from build123d import *

# Parameters (mm, degrees)
CUT_EXTRUDE1_DEPTH       = 22.365860619
CUT_EXTRUDE1_DEPTH_BACK  = 22.365860619
SKETCH2_R                = 1.5
SKETCH3_W                = 9.16515139
SKETCH3_H                = 1.7
CUT_EXTRUDE2_DEPTH       = 21.310096204
FILLET1_R                = 0.4
BOSS_EXTRUDE1_START      = 19.2405
SKETCH4_R                = 6.5
SKETCH4_R_2              = 3
BOSS_EXTRUDE1_DEPTH      = 19.2405
CHAMFER1_SIZE            = 1.5
CHAMFER2_SIZE            = 0.5
FILLET2_R                = 0.5
CUT_EXTRUDE3_START       = -19.2405
CUT_EXTRUDE3_OUTLINE_R   = 7.963373885
CUT_EXTRUDE3_OUTLINE_R_2 = 3
CUT_EXTRUDE3_DEPTH       = 19.2405
SKETCH6_R                = 3.5
CUT_EXTRUDE4_DEPTH       = 10
CHAMFER3_SIZE            = 0.5
SKETCH7_R                = 10.7
CUT_EXTRUDE5_DEPTH       = 10
CUT_EXTRUDE6_START       = 5.5
CUT_EXTRUDE6_DEPTH       = 1.7
CHAMFER5_SIZE            = 1


# Read off the part's stored shape, not the designer's step: Cut-Extrude3
with BuildPart() as part:
    # Sketch1 → Revolve1 (revolve)
    with BuildSketch(Plane.XY, mode=Mode.PRIVATE) as revolve1_sk:
        Polygon((-12, 12.5), (0, 12.5), (6, 12.5), (6, 10), (6, 3), (-2, 3), (-2, 10.2), (-12, 10.2), align=None)
    revolve(revolve1_sk.sketch.rotate(Axis((88.99, 0, 0), (-1, 0, 0)), 90), axis=Axis((88.99, 0, 0), (-1, 0, 0)))

    # Sketch2 → Cut-Extrude1 (cut, two sides: drawn at the far end of the back side and taken through both)
    with BuildSketch(Plane(origin=(0, 0, 0), x_dir=(1, 0, 0), z_dir=(0, 1, 0)).offset(-CUT_EXTRUDE1_DEPTH_BACK)):
        with Locations(Location((3, 0, 0), (0, 0, 90))):
            Circle(SKETCH2_R)
    extrude(amount=CUT_EXTRUDE1_DEPTH + CUT_EXTRUDE1_DEPTH_BACK, mode=Mode.SUBTRACT)

    # Sketch3 → Cut-Extrude2 (cut, through all)
    with BuildSketch(Plane.ZY.offset(2)):
        with Locations((-4.582575695, 9.35)):
            Rectangle(SKETCH3_W, SKETCH3_H)
    extrude(amount=CUT_EXTRUDE2_DEPTH, mode=Mode.SUBTRACT)

    # Fillet1
    fillet1_edges = [part.edges().sort_by_distance(p)[0] for p in [
        (-7, 8.5, -5.638262144),
        (-7, 10.2, -7.22564876),
        (-7, 8.5, -9.16515139),
    ]]
    fillet(fillet1_edges, radius=FILLET1_R)

    # Sketch4 → Boss-Extrude1 (add)
    with BuildSketch(Plane.ZY.offset(2).offset(BOSS_EXTRUDE1_START)):
        Circle(SKETCH4_R)
        with Locations(Location((0, 0, 0), (0, 0, 180))):
            Circle(SKETCH4_R_2, mode=Mode.SUBTRACT)
    extrude(amount=-BOSS_EXTRUDE1_DEPTH)

    # Chamfer1
    chamfer1_edges = [part.edges().sort_by_distance(p)[0] for p in [
        (-21.2405, 0, -6.5),
        (-21.2405, 0, 3),
    ]]
    chamfer(chamfer1_edges, length=CHAMFER1_SIZE)

    # Chamfer2
    chamfer2_edges = [part.edges().sort_by_distance(p)[0] for p in [
        (6, 0, 3),
    ]]
    chamfer(chamfer2_edges, length=CHAMFER2_SIZE)

    # Fillet2
    # the kernel refuses this fillet: 0.5 mm, written as the material it adds along each edge
    with BuildSketch(Plane(origin=(-2, 0, 0), x_dir=(0, 0.7641509433962261, -0.6450374684517619), z_dir=(0, 0.6450374684517619, 0.7641509433962261))) as fillet2_piece_1:
        with BuildLine():
            CenterArc((10.2 - FILLET2_R, FILLET2_R), FILLET2_R, 270, 90)
            Line((10.2, FILLET2_R), (10.2, 0))
            Line((10.2, 0), (10.2 - FILLET2_R, 0))
        make_face()
    revolve(axis=Axis((-2, 0, 0), (-1, 0, 0)), revolution_arc=319.831515217)
    with BuildSketch(Plane(origin=(-2, 10.2, 0), x_dir=(0, -1, 0), z_dir=(0, 0, -1))) as fillet2_piece_2:
        with BuildLine():
            CenterArc((FILLET2_R, FILLET2_R), FILLET2_R, 180, 90)
            Line((0, FILLET2_R), (0, 0))
            Line((0, 0), (FILLET2_R, 0))
        make_face()
    extrude(amount=5.835237784)
    with BuildSketch(Plane(origin=(-2, 8.5, -8.988882022), x_dir=(0, 1, 0), z_dir=(0, 0, 1))) as fillet2_piece_3_section:
        with BuildLine():
            CenterArc((FILLET2_R, FILLET2_R), FILLET2_R, 180, 90)
            Line((0, FILLET2_R), (0, 0))
            Line((0, 0), (FILLET2_R, 0))
        make_face()
    fillet2_piece_3 = extrude(amount=2.151484856, mode=Mode.PRIVATE)
    fillet2_piece_3 = fillet2_piece_3 & Plane(origin=(-2.112337318, 0, 0), x_dir=(0, 0, -1), z_dir=(1, 0, 0)) * Cylinder(12.5, 7, mode=Mode.PRIVATE)
    add(fillet2_piece_3)
    with BuildSketch(Plane(origin=(-2, 8.1, -6.837397166), x_dir=(0, -0.7641509433962268, 0.6450374684517612), z_dir=(0, -0.6450374684517612, -0.7641509433962268))) as fillet2_piece_4:
        with BuildLine():
            CenterArc((0.4 + FILLET2_R, FILLET2_R), FILLET2_R, 180, 90)
            Line((0.4, FILLET2_R), (0.4, 0))
            Line((0.4, 0), (0.4 + FILLET2_R, 0))
        make_face()
    revolve(axis=Axis((-2, 8.1, -6.837397166), (-1, 0, 0)), revolution_arc=139.831515217)
    with BuildSketch(Plane(origin=(-2, 8.1, -8.988882022), x_dir=(0, -0.6813941617388248, 0.7319166594280009), z_dir=(0, 0.7319166594280009, 0.6813941617388248))) as fillet2_piece_5_section:
        with BuildLine():
            CenterArc((0.4 + FILLET2_R, -FILLET2_R), FILLET2_R, 90, 90)
            Line((0.4, -FILLET2_R), (0.4, 0))
            Line((0.4, 0), (0.4 + FILLET2_R, 0))
        make_face()
    fillet2_piece_5 = revolve(axis=Axis((-2, 8.1, -8.988882022), (1, 0, 0)), revolution_arc=227.047315948, mode=Mode.PRIVATE)
    fillet2_piece_5 = fillet2_piece_5 & Plane(origin=(-2.20433756, 0, 0), x_dir=(0, 0, -1), z_dir=(1, 0, 0)) * Cylinder(12.5, 4, mode=Mode.PRIVATE)
    add(fillet2_piece_5)
    with BuildSketch(Plane(origin=(-2, 10.6, -5.835237784), x_dir=(0, -0.8696656127523182, 0.49364128878785535), z_dir=(0, -0.49364128878785535, -0.8696656127523182))) as fillet2_piece_6_section:
        with BuildLine():
            CenterArc((0.4 + FILLET2_R, FILLET2_R), FILLET2_R, 180, 90)
            Line((0.4 + FILLET2_R, 0), (0.4, 0))
            Line((0.4, 0), (0.4, FILLET2_R))
        make_face()
    fillet2_piece_6 = revolve(axis=Axis((-2, 10.6, -5.835237784), (-1, 0, 0)), revolution_arc=330.419804772, mode=Mode.PRIVATE)
    fillet2_piece_6 = fillet2_piece_6 & Plane(origin=(-2.048284791, 0, 0), x_dir=(0, 0, -1), z_dir=(1, 0, 0)) * Cylinder(12.5, 4, mode=Mode.PRIVATE)
    add(fillet2_piece_6)
    with BuildSketch(Plane(origin=(-2, 0, 0), x_dir=(0, 0, 1), z_dir=(0, -1, 0))) as fillet2_piece_7:
        with BuildLine():
            CenterArc((6.5 + FILLET2_R, FILLET2_R), FILLET2_R, 180, 90)
            Line((6.5, FILLET2_R), (6.5, 0))
            Line((6.5, 0), (6.5 + FILLET2_R, 0))
        make_face()
    revolve(axis=Axis((-2, 0, 0), (-1, 0, 0)))

    # Cut-Extrude3 outline → Cut-Extrude3 (cut)
    with BuildSketch(Plane.ZY.offset(21.2405).offset(CUT_EXTRUDE3_START)):
        Circle(CUT_EXTRUDE3_OUTLINE_R)
        Circle(CUT_EXTRUDE3_OUTLINE_R_2, mode=Mode.SUBTRACT)
    extrude(amount=CUT_EXTRUDE3_DEPTH, mode=Mode.SUBTRACT)

    # Sketch6 → Cut-Extrude4 (cut)
    with BuildSketch(Plane(origin=(6, 0, 0), x_dir=(0, 0, -1), z_dir=(1, 0, 0))):
        Circle(SKETCH6_R)
    extrude(amount=-CUT_EXTRUDE4_DEPTH, mode=Mode.SUBTRACT)

    # Chamfer3
    chamfer3_edges = [part.edges().sort_by_distance(p)[0] for p in [
        (6, 0, 3.5),
    ]]
    chamfer(chamfer3_edges, length=CHAMFER3_SIZE)

    # Sketch7 → Cut-Extrude5 (cut)
    with BuildSketch(Plane.ZY.offset(12)):
        Circle(SKETCH7_R)
    extrude(amount=-CUT_EXTRUDE5_DEPTH, mode=Mode.SUBTRACT)

    # Sketch8 → Cut-Extrude6 (cut)
    with BuildSketch(Plane(origin=(0, 0, 0), x_dir=(1, 0, 0), z_dir=(0, 1, 0)).offset(CUT_EXTRUDE6_START)):
        Polygon((0.2, 1.616580754), (0.2, -1.616580754), (0.2, -2.424871131), (3, -3.233161507), (4.318553482, -3.233161507), (8.377038533, -3.233161507), (8.377038533, 3.233161507), (4.318553482, 3.233161507), (3, 3.233161507), (0.2, 2.424871131), align=None)
    cut_extrude6 = extrude(amount=CUT_EXTRUDE6_DEPTH, mode=Mode.SUBTRACT)

    # Chamfer5
    chamfer5_edges = [part.edges().sort_by_distance(p)[0] for p in [
        (6, 0, 12.5),
    ]]
    chamfer(chamfer5_edges, length=CHAMFER5_SIZE)

    # Mirror1: Cut-Extrude6 across plane
    add(cut_extrude6.mirror(Plane.ZX), mode=Mode.SUBTRACT)


solid = part.part
The model under review builds one solid part; all positions refer to its coordinate system, in mm. A direction names the side the tool comes from. Coordinates: 2 decimals unless noted, no trailing zeros. Loops run counter-clockwise (first coordinate to the right, second up) from the corner with the lowest first, then second, coordinate; pieces in that order, holes last. Notation, with made-up numbers: (-36, 89) -> (-10, 89) arc R14 ccw to (-10, 110) -> close; hole circle Ø2 at (35, -13). An arc over 180 degrees is marked (long way). Use a Markdown table: item, result. Add a question column.
1. Add section D-D on x = -1. Write out the cut boundary in (y, z).
2. To check wall thickness, follow line 1 (X direction, y = -11.4, z = 0); line 2 (X direction, y = -10.35, z = 0); line 3 (Y direction, x = 0.5, z = -1.25). State the ranges of each line that lie inside material, in increasing order.
3. Clearance check with flat-ended pins moving along their axes: pin 1 Ø3 at (x, z) = (-8, 9) entering from +Y; pin 2 Ø1 at (x, y) = (-2.5, 6) entering from +Z (3 decimals); pin 3 Ø0.8 at (x, y) = (5, -6.5) entering from +Z. State where each tip first meets the part, or that it passes through.
4. Machinability: for faces 4 (the face through (-2, 3, -3)), 5 (the face through (-7, 10.2, -5)), 6 (the face through (0.2, 6, 0)), which of the approach directions +Z, -Z, +X, -X, +Y, -Y give a long, thin tool a straight path to every point of the face, cutting with its end or side? Answer none if there is none.
5. Add section C-C on z = 0. Give the number of separate pieces and of enclosed holes in the cut face, plus the area to 3 significant figures.
6. Add section B-B on x = 3.5. Write out the cut boundary in (y, z).
7. Add section A-A on y = 0. Write out the cut boundary in (x, z), plus the area to 3 significant figures.
8. Draft analysis for pull direction X (two halves, no side actions). For faces 1 (the face through (4, -6, 3.233)), 2 (the face through (0.2, -6, 0)), 3 (the face through (2.55, 4.31, -1.43)), state which applies: pulls with the +X half, pulls with the -X half, needs draft (parallel to the pull), parting line crosses it, or undercut.
Returned:
| question | item | result |
|---|---|---|
| 1 | outline | circle Ø25 at (0, 0); hole circle Ø7 at (0, 0) |
| 2 | line 1 | x = -12 to 1.5, 4.5 to 6 |
| 2 | line 2 | x = -2 to 1.5, 4.5 to 6 |
| 2 | line 3 | y = -12.44 to -7.2, -5.5 to -3.27, 3.27 to 5.5, 7.2 to 12.44 |
| 3 | pin 1 | stops at y = 10 |
| 3 | pin 2 | stops at z = 11.225 |
| 3 | pin 3 | stops at z = 10.91 |
| 4 | face 4 | -X |
| 4 | face 5 | -Z, -X |
| 4 | face 6 | +X |
| 5 | separate pieces | 6 |
| 5 | enclosed holes | 0 |
| 5 | area | 115 mm² |
| 6 | outline | (-12.42, -1.41) arc R12.5 ccw to (12.42, -1.41) -> (7.2, -1.41) -> (7.2, -3.23) -> (5.5, -3.23) -> (5.5, -1.41) -> (3.2, -1.41) arc R3.5 cw to (-3.2, -1.41) -> (-5.5, -1.41) -> (-5.5, -3.23) -> (-7.2, -3.23) -> (-7.2, -1.41) -> close; (-12.42, 1.41) -> (-7.2, 1.41) -> (-7.2, 3.23) -> (-5.5, 3.23) -> (-5.5, 1.41) -> (-3.2, 1.41) arc R3.5 cw to (3.2, 1.41) -> (5.5, 1.41) -> (5.5, 3.23) -> (7.2, 3.23) -> (7.2, 1.41) -> (12.42, 1.41) arc R12.5 ccw to start |
| 7 | outline | (-12, -12.5) -> (5, -12.5) -> (6, -11.5) -> (6, -4) -> (5.5, -3.5) -> (-2, -3.5) -> (-2, -10.7) -> (-12, -10.7) -> close; (-12, 10.7) -> (-2, 10.7) -> (-2, 3.5) -> (5.5, 3.5) -> (6, 4) -> (6, 11.5) -> (5, 12.5) -> (-12, 12.5) -> close |
| 7 | area | 179 mm² |
| 8 | face 1 | needs draft |
| 8 | face 2 | pulls with the +X half |
| 8 | face 3 | undercut |
